Input: part model. Units: mm. Frame: model coordinates. Round coordinates to 2 decimals unless told otherwise and drop trailing zeros. Loops run counter-clockwise (first coordinate to the right, second up) from the corner with the lowest first, then second, coordinate; pieces in that order, holes last. Notation, with made-up numbers: (79, 36.25) - (127, 36.25) arc R15 cw to (127, 52.25) - close; hole circle Ø4 at (11.5, 62.5). An arc over 180 degrees is marked (long way). Use CSV: the item, a comma, the result in double quotes. Start each with the question number.
1. Cut plane B-B (z = -30). Return loops of the section in (x, y), and give its area (3 significant figures).
2. Pull-direction query (Z, two-part tool) for faces 1 (the flat face through (433, 0, -25)), 2 (the flat face through (433, -2.032, -26)); classes: +Z half, -Z half, draft (parallel to the pull), parting line (faces both ways), or undercut.
3. Cut plane A-A (x = 806.5). Return loops of the section in (y, z) (1 decimal), and give its area (3 significant figures).
4. Material intervals for probe 1 along Y at (x, z) = (721, -23.5); probe 2 along Z at (x, y) = (637, -4); probe 3 along Z at (x, y) = (517, -5.5), sorted ascending. Write a range as from..to.
5. Pin query (flat end, axial travel): P1, Ø3, axis at x = 680.5, z = -25.5, coming from the -Y side; P2, Ø2, axis at x = 347, y = -5, coming from the -Z side; P3, Ø4, axis at x = 616.5, y = -3.5, coming from the +Z side. Return the tip coordinate at first contact, or that it passes through.
Autodesk Inventor part; units mm, degrees
ref_plane "YZ Plane" through (0, 0, 0) normal (1, 0, 0) x (0, 1, 0)
ref_plane "XZ Plane" through (0, 0, 0) normal (0, 1, 0) x (-1, 0, 0)
ref_plane "XY Plane" through (0, 0, 0) normal (0, 0, 1) x (1, 0, 0)
sketch "Sketch1" plane through (0, 0, 0) normal (1, 0, 0) x (0, 1, 0)
  line L0 (0, -0.4446) -> (0, -50.3554)
  line L1 (-0.4178, -50.9521) -> (-9.1295, -54.1229)
  line L2 (-9.8331, -53.9343) -> (-12.8126, -50.3834)
  line L3 (-0.4178, 0.1521) -> (-9.1295, 3.3229)
  line L4 (-9.8331, 3.1343) -> (-12.8126, -0.4166)
  line L5 (-11.256, -49.0773) -> (-9.1911, -51.5382)
  line L6 (-8.4874, -51.7268) -> (-2.4498, -49.5293)
  line L7 (-2.032, -48.9325) -> (-2.032, -1.8675)
  line L8 (-2.4498, -1.2707) -> (-8.4874, 0.9268)
  line L9 (-9.1911, 0.7382) -> (-11.256, -1.7227)
  line L10 (-12.8126, -0.4166) -> (-11.256, -1.7227)
  line L11 (-11.256, -49.0773) -> (-12.8126, -50.3834)
  arc A0 (0, -0.4446) -> (-0.4178, 0.1521) centre (-0.635, -0.4446) ccw
  arc A1 (-2.032, -1.8675) -> (-2.4498, -1.2707) centre (-2.667, -1.8675) ccw
  arc A2 (-9.1295, 3.3229) -> (-9.8331, 3.1343) centre (-9.3466, 2.7261) ccw
  arc A3 (-8.4874, 0.9268) -> (-9.1911, 0.7382) centre (-8.7046, 0.3301) ccw
  arc A4 (-2.4498, -49.5293) -> (-2.032, -48.9325) centre (-2.667, -48.9325) ccw
  arc A5 (-0.4178, -50.9521) -> (0, -50.3554) centre (-0.635, -50.3554) ccw
  arc A6 (-9.1911, -51.5382) -> (-8.4874, -51.7268) centre (-8.7046, -51.1301) ccw
  arc A7 (-9.8331, -53.9343) -> (-9.1295, -54.1229) centre (-9.3466, -53.5261) ccw
  point P0 (0, 0)
  point P1 (0, -50.8)
  point P2 (-9.5473, -54.2749)
  point P3 (-9.5473, 3.4749)
  dimension "d0" = 50.8
  dimension "d1" = 10.16
  dimension "d2" = 5.08
  dimension "d3" = 110
  dimension "d4" = 110
  dimension "d5" = 10.16
  dimension "d6" = 5.08
  dimension "d7" = 110
  dimension "d8" = 110
  dimension "d9" = 2.032
  dimension "d10" = 0.635
extrude "Extrusion1" add sketch "Sketch1" along normal blind 878.84
properties part number "the outside slider part"
Established:
1,outline,"(0, -2.03) - (878.84, -2.03) - (878.84, 0) - (0, 0) - close"
1,area,"1,790 mm2"
2,face 1,"draft"
2,face 2,"undercut"
3,outline,"(-12.8, -50.4) - (-9.8, -53.9) arc R0.6 ccw to (-9.1, -54.1) - (-0.4, -51) arc R0.6 ccw to (0, -50.4) - (0, -0.4) arc R0.6 ccw to (-0.4, 0.2) - (-9.1, 3.3) arc R0.6 ccw to (-9.8, 3.1) - (-12.8, -0.4) - (-11.3, -1.7) - (-9.2, 0.7) arc R0.6 cw to (-8.5, 0.9) - (-2.4, -1.3) arc R0.6 cw to (-2, -1.9) - (-2, -48.9) arc R0.6 cw to (-2.4, -49.5) - (-8.5, -51.7) arc R0.6 cw to (-9.2, -51.5) - (-11.3, -49.1) - close"
3,area,"154 mm2"
4,probe 1,"y = -2.03..0"
4,probe 2,"z = -52.26..-50.09, -0.71..1.46"
4,probe 3,"z = -52.8..-50.64, -0.16..2"
5,P1,"stops at y = -2.03"
5,P2,"stops at z = -52.98"
5,P3,"stops at z = 2"
